Build history of the part. All positions in model axes, mm. Round coordinates to 2 decimals unless told otherwise and drop trailing zeros. Write each loop counter-clockwise with the first axis right and the second up, starting at its lowest first coordinate (ties: lowest second). Pieces come first, ordered by that corner, then holes.
1) Saw through at C-C (z = 1.85). State how many separate pieces and enclosed holes the cut face has, plus the area to 3 significant figures.
2) Flat gauge pins, fed straight in: pin 1 (1 mm diameter, centred on x = -47.5, y = -19.5, fed in from -Z); pin 2 (3 mm diameter, centred on x = -36.51, y = -9.09, fed in from -Z). Where does each tip first touch, or does it go through?
3) Saw through at A-A (x = -27.5). Write the cut outline in (y, z).
4) Pull direction Y, two halves, no side cores. Call faces 1 (the cylindrical face through (-53.156, 29.649, 2.535)), 2 (the cylindrical face through (-35.353, 21.43, 2.465)), 3 (the flat face through (-21, -77.344, 2)): +Y half, -Y half, draft (parallel to the pull), parting line (faces both ways), or undercut.
5) Saw through at B-B (y = 13.5). Write the cut outline in (x, z), plus the area to 3 significant figures.
6) Wall check: probe 1 along Y at (x, z) = (7, 4.7); probe 2 along X at (y, z) = (-69.5, 2.8); probe 3 along Y at (x, z) = (-23.5, 3.15). Give the ranges that are in metal, low to high.
from build123d import *

# Parameters (mm, degrees)
SKETCH1_W           = 70
SKETCH1_H           = 110
SKETCH1_R           = 2.5
SKETCH1_R_2         = 12.5
SKETCH1_R_3         = 1.25
BOSS_EXTRUDE1_DEPTH = 5
FILLET1_R           = 10


with BuildPart() as part:
    # Sketch1 → Boss-Extrude1 (new body)
    with BuildSketch(Plane.XY):
        with Locations((-21.007524629, -22.344146878)):
            Rectangle(SKETCH1_W, SKETCH1_H)
        with Locations((-48.507524629, -19.844146878)):
            Circle(SKETCH1_R, mode=Mode.SUBTRACT)
        with Locations((6.492475371, -19.844146878)):
            Circle(SKETCH1_R, mode=Mode.SUBTRACT)
        with Locations((-48.507524629, -69.844146878)):
            Circle(SKETCH1_R, mode=Mode.SUBTRACT)
        with Locations((6.492475371, -69.844146878)):
            Circle(SKETCH1_R, mode=Mode.SUBTRACT)
        with Locations((-21.007524629, 6.405853122)):
            Circle(SKETCH1_R_2, mode=Mode.SUBTRACT)
        with Locations((-36.507524629, 21.908578371)):
            Circle(SKETCH1_R_3, mode=Mode.SUBTRACT)
        with Locations((-5.507524629, 21.903128352)):
            Circle(SKETCH1_R_3, mode=Mode.SUBTRACT)
        with Locations((-5.507524629, -9.096872127)):
            Circle(SKETCH1_R_3, mode=Mode.SUBTRACT)
        with Locations((-36.507524629, -9.091422108)):
            Circle(SKETCH1_R_3, mode=Mode.SUBTRACT)
    extrude(amount=BOSS_EXTRUDE1_DEPTH)

    # Fillet1
    fillet1_edges = [part.edges().sort_by_distance(p)[0] for p in [
        (-56.007524629, 32.655853122, 2.5),
        (13.992475371, 32.655853122, 2.5),
        (13.992475371, -77.344146878, 2.5),
        (-56.007524629, -77.344146878, 2.5),
    ]]
    fillet(fillet1_edges, radius=FILLET1_R)


solid = part.part
Evaluation:
1. separate pieces: 1
1. enclosed holes: 9
1. area: 7,030 mm2
2. pin 1: passes through
2. pin 2: stops at z = 0
3. outline: (-77.34, 0) - (-4.28, 0) - (-4.28, 5) - (-77.34, 5) - close; (17.09, 0) - (32.66, 0) - (32.66, 5) - (17.09, 5) - close
4. face 1: +Y half
4. face 2: undercut
4. face 3: -Y half
5. outline: (-56.01, 0) - (-31.3, 0) - (-31.3, 5) - (-56.01, 5) - close; (-10.72, 0) - (13.99, 0) - (13.99, 5) - (-10.72, 5) - close
5. area: 247 mm2
6. probe 1: y = -76.88 to -72.29, -67.4 to -22.29, -17.4 to 32.19
6. probe 2: x = -55.77 to -50.98, -46.03 to 4.02, 8.97 to 13.76
6. probe 3: y = -77.34 to -5.84, 18.65 to 32.66
